The listing builds one solid part. Answer for the finished solid, in the listing's coordinates (mm). Face numbers are marked on the shaded views. A direction names the side the tool comes from. Coordinates: 2 decimals unless noted, no trailing zeros. Order: outer loops, then holes, each group sorted by start corner. A loop starts at its lowest first (then second) coordinate and runs counter-clockwise, first axis right, second up. Notation, with made-up numbers: M 58,42 L 95,42 A34 cw 95,74 Z; hole C 1,56 d9. An arc over 180 degrees is marked long. One line per item, written item: value. Start each with the question number.
Q1. The part is cut by section B-B on z = -55. Give the vertices of the cut face in (x, y), then the cut area to 3 significant figures.
Q2. Each of these flat-tipped pins is pushed along its axis until it touches: pin 1 Ø1.5 at (x, z) = (142.5, -13.5) entering from +Y; pin 2 Ø1.5 at (x, y) = (142.5, -3) entering from -Z; pin 3 Ø2.5 at (x, y) = (142.5, -3) entering from +Z. Where does it stop, or does it pass through?
Q3. The part is cut by section A-A on x = 144. Give the vertices of the cut face in (y, z), then the cut area to 3 significant figures.
Q4. Straight lines are drawn through the part: line 1 along Z through (x, y) = (141.6, -11); line 2 along Y through (x, z) = (141.25, -58); line 3 along Y through (x, z) = (144.05, -38). For each, find the intervals that lie inside material, in ascending order. Write a range as [from, to].
Q5. The part is cut by section C-C on y = -40. Give the vertices of the cut face in (x, z), then the cut area to 3 significant figures.
Q6. For the marked faces 1, 2 and 3, determine the directions among +Z, -Z, +X, -X, +Y, -Y from which every point of the face is accessible in a straight line to the end or side of a thin tool.
```python
from build123d import *

# Parameters (mm, degrees)
BODY_MOVE_COPY1_START         = -65
BODY_MOVE_COPY1_OUTLINE_W     = 5.1
BODY_MOVE_COPY1_OUTLINE_H     = 30.1
BODY_MOVE_COPY1_OUTLINE_R     = 2.6
BODY_MOVE_COPY1_OUTLINE_R_2   = 3.1
BODY_MOVE_COPY1_OUTLINE_R_3   = 1.55
BODY_MOVE_COPY1_OUTLINE_W_2   = 30.5
BODY_MOVE_COPY1_OUTLINE_H_2   = 14.5
BODY_MOVE_COPY1_DEPTH         = 5
BODY_MOVE_COPY1_START_2       = -5
BODY_MOVE_COPY1_2_OUTLINE_W   = 10
BODY_MOVE_COPY1_2_OUTLINE_H   = 5.2
BODY_MOVE_COPY1_2_OUTLINE_R   = 1.6
BODY_MOVE_COPY1_2_OUTLINE_W_2 = 5.1
BODY_MOVE_COPY1_2_OUTLINE_H_2 = 30.1
BODY_MOVE_COPY1_2_DEPTH       = 5
BOSS_EXTRUDE2_DEPTH           = 5


# Read off the part's stored shape, not the designer's step: Body-Move/Copy1
with BuildPart() as part:
    # Body-Move/Copy1 outline → Body-Move/Copy1 (new body)
    with BuildSketch(Plane.XY.offset(BODY_MOVE_COPY1_START)):
        Polygon((24.9, -310), (24.9, -305), (100.2, -305), (100.2, -310), (150, -310), (150, -5), (10.65, -5), (10.65, 0), (-10.65, 0), (-10.65, -5), (-150, -5), (-150, -310), (-100.2, -310), (-100.2, -305), (-24.9, -305), (-24.9, -310), align=None)
        with Locations((-143.45, -280)):
            Rectangle(BODY_MOVE_COPY1_OUTLINE_W, BODY_MOVE_COPY1_OUTLINE_H, mode=Mode.SUBTRACT)
        with Locations((-90, -157.5)):
            Circle(BODY_MOVE_COPY1_OUTLINE_R, mode=Mode.SUBTRACT)
        with Locations((-60, -157.5)):
            Circle(BODY_MOVE_COPY1_OUTLINE_R, mode=Mode.SUBTRACT)
        with Locations((143.45, -280)):
            Rectangle(BODY_MOVE_COPY1_OUTLINE_W, BODY_MOVE_COPY1_OUTLINE_H, mode=Mode.SUBTRACT)
        with Locations((65, -157.5)):
            Circle(BODY_MOVE_COPY1_OUTLINE_R_2, mode=Mode.SUBTRACT)
        with Locations((85, -157.5)):
            Circle(BODY_MOVE_COPY1_OUTLINE_R_2, mode=Mode.SUBTRACT)
        with Locations((-90, -137.5)):
            Circle(BODY_MOVE_COPY1_OUTLINE_R_3, mode=Mode.SUBTRACT)
        with Locations((-60, -137.5)):
            Circle(BODY_MOVE_COPY1_OUTLINE_R_3, mode=Mode.SUBTRACT)
        with Locations((-75, -100.25)):
            Rectangle(BODY_MOVE_COPY1_OUTLINE_W_2, BODY_MOVE_COPY1_OUTLINE_H_2, mode=Mode.SUBTRACT)
        with Locations((-143.45, -30)):
            Rectangle(BODY_MOVE_COPY1_OUTLINE_W, BODY_MOVE_COPY1_OUTLINE_H, mode=Mode.SUBTRACT)
        with Locations((143.45, -30)):
            Rectangle(BODY_MOVE_COPY1_OUTLINE_W, BODY_MOVE_COPY1_OUTLINE_H, mode=Mode.SUBTRACT)
    extrude(amount=BODY_MOVE_COPY1_DEPTH)


with BuildPart() as body_2:
    # Body-Move_Copy1 2 outline → Body-Move_Copy1 2 (new body)
    with BuildSketch(Plane(origin=(0, 0, 0), x_dir=(1, 0, 0), z_dir=(0, 1, 0)).offset(BODY_MOVE_COPY1_START_2)):
        with BuildLine():
            ThreePointArc((-95, -65), (-93.535533906, -61.464466094), (-90, -60))
            Line((-90, -60), (90, -60))
            ThreePointArc((90, -60), (93.535533906, -61.464466094), (95, -65))
            Line((95, -65), (95, -70))
            ThreePointArc((95, -70), (96.464466094, -73.535533906), (100, -75))
            Line((100, -75), (115, -75))
            ThreePointArc((115, -75), (118.535533906, -73.535533906), (120, -70))
            Line((120, -70), (120, -60))
            Line((120, -60), (145.606601718, -34.393398282))
            ThreePointArc((145.606601718, -34.393398282), (148.858192988, -29.52704805), (150, -23.786796564))
            Line((150, -23.786796564), (150, 65))
            Line((150, 65), (10.75, 65))
            Line((10.75, 65), (10.75, 60))
            Line((10.75, 60), (-10.75, 60))
            Line((-10.75, 60), (-10.75, 65))
            Line((-10.75, 65), (-150, 65))
            Line((-150, 65), (-150, -23.786796564))
            ThreePointArc((-150, -23.786796564), (-148.858192988, -29.52704805), (-145.606601718, -34.393398282))
            Line((-145.606601718, -34.393398282), (-120, -60))
            Line((-120, -60), (-120, -70))
            ThreePointArc((-120, -70), (-118.535533906, -73.535533906), (-115, -75))
            Line((-115, -75), (-100, -75))
            ThreePointArc((-100, -75), (-96.464466094, -73.535533906), (-95, -70))
            Line((-95, -70), (-95, -65))
        make_face()
        with Locations((-107.5, -67.5)):
            Rectangle(BODY_MOVE_COPY1_2_OUTLINE_W, BODY_MOVE_COPY1_2_OUTLINE_H, mode=Mode.SUBTRACT)
        with Locations((-110, -52.5)):
            Circle(BODY_MOVE_COPY1_2_OUTLINE_R, mode=Mode.SUBTRACT)
        with Locations((-5, -52.5)):
            Circle(BODY_MOVE_COPY1_2_OUTLINE_R, mode=Mode.SUBTRACT)
        with Locations((5, -52.5)):
            Circle(BODY_MOVE_COPY1_2_OUTLINE_R, mode=Mode.SUBTRACT)
        with Locations((107.5, -67.5)):
            Rectangle(BODY_MOVE_COPY1_2_OUTLINE_W, BODY_MOVE_COPY1_2_OUTLINE_H, mode=Mode.SUBTRACT)
        with Locations((110, -52.5)):
            Circle(BODY_MOVE_COPY1_2_OUTLINE_R, mode=Mode.SUBTRACT)
        with Locations((-143.45, 35)):
            Rectangle(BODY_MOVE_COPY1_2_OUTLINE_W_2, BODY_MOVE_COPY1_2_OUTLINE_H_2, mode=Mode.SUBTRACT)
        with Locations((-110, 52.5)):
            Circle(BODY_MOVE_COPY1_2_OUTLINE_R, mode=Mode.SUBTRACT)
        with Locations((-5, 52.5)):
            Circle(BODY_MOVE_COPY1_2_OUTLINE_R, mode=Mode.SUBTRACT)
        with BuildLine():
            Line((131.606601718, -30.178932188), (115.267766953, -46.517766953))
            ThreePointArc((115.267766953, -46.517766953), (114.456708581, -47.059698831), (113.5, -47.25))
            Line((113.5, -47.25), (107.75, -47.25))
            ThreePointArc((107.75, -47.25), (105.982233047, -47.982233047), (105.25, -49.75))
            Line((105.25, -49.75), (105.25, -53.5))
            ThreePointArc((105.25, -53.5), (104.517766953, -55.267766953), (102.75, -56))
            Line((102.75, -56), (13.25, -56))
            ThreePointArc((13.25, -56), (11.482233047, -55.267766953), (10.75, -53.5))
            Line((10.75, -53.5), (10.75, -49.75))
            ThreePointArc((10.75, -49.75), (10.017766953, -47.982233047), (8.25, -47.25))
            Line((8.25, -47.25), (-8.25, -47.25))
            ThreePointArc((-8.25, -47.25), (-10.017766953, -47.982233047), (-10.75, -49.75))
            Line((-10.75, -49.75), (-10.75, -53.5))
            ThreePointArc((-10.75, -53.5), (-11.482233047, -55.267766953), (-13.25, -56))
            Line((-13.25, -56), (-102.75, -56))
            ThreePointArc((-102.75, -56), (-104.517766953, -55.267766953), (-105.25, -53.5))
            Line((-105.25, -53.5), (-105.25, -49.75))
            ThreePointArc((-105.25, -49.75), (-105.982233047, -47.982233047), (-107.75, -47.25))
            Line((-107.75, -47.25), (-113.5, -47.25))
            ThreePointArc((-113.5, -47.25), (-115.267766953, -46.517766953), (-116, -44.75))
            Line((-116, -44.75), (-116, 44.75))
            ThreePointArc((-116, 44.75), (-115.267766953, 46.517766953), (-113.5, 47.25))
            Line((-113.5, 47.25), (-107.75, 47.25))
            ThreePointArc((-107.75, 47.25), (-105.982233047, 47.982233047), (-105.25, 49.75))
            Line((-105.25, 49.75), (-105.25, 53.5))
            ThreePointArc((-105.25, 53.5), (-104.517766953, 55.267766953), (-102.75, 56))
            Line((-102.75, 56), (-13.25, 56))
            ThreePointArc((-13.25, 56), (-11.482233047, 55.267766953), (-10.75, 53.5))
            Line((-10.75, 53.5), (-10.75, 49.75))
            ThreePointArc((-10.75, 49.75), (-10.017766953, 47.982233047), (-8.25, 47.25))
            Line((-8.25, 47.25), (8.25, 47.25))
            ThreePointArc((8.25, 47.25), (10.017766953, 47.982233047), (10.75, 49.75))
            Line((10.75, 49.75), (10.75, 53.5))
            ThreePointArc((10.75, 53.5), (11.482233047, 55.267766953), (13.25, 56))
            Line((13.25, 56), (102.75, 56))
            ThreePointArc((102.75, 56), (104.517766953, 55.267766953), (105.25, 53.5))
            Line((105.25, 53.5), (105.25, 49.75))
            ThreePointArc((105.25, 49.75), (105.982233047, 47.982233047), (107.75, 47.25))
            Line((107.75, 47.25), (113.5, 47.25))
            ThreePointArc((113.5, 47.25), (115.267766953, 47.982233047), (116, 49.75))
            Line((116, 49.75), (116, 53.5))
            ThreePointArc((116, 53.5), (116.732233047, 55.267766953), (118.5, 56))
            Line((118.5, 56), (133.5, 56))
            ThreePointArc((133.5, 56), (135.267766953, 55.267766953), (136, 53.5))
            Line((136, 53.5), (136, -19.57233047))
            ThreePointArc((136, -19.57233047), (134.858192988, -25.312581956), (131.606601718, -30.178932188))
        make_face(mode=Mode.SUBTRACT)
        with Locations((5, 52.5)):
            Circle(BODY_MOVE_COPY1_2_OUTLINE_R, mode=Mode.SUBTRACT)
        with Locations((143.45, 35)):
            Rectangle(BODY_MOVE_COPY1_2_OUTLINE_W_2, BODY_MOVE_COPY1_2_OUTLINE_H_2, mode=Mode.SUBTRACT)
        with Locations((110, 52.5)):
            Circle(BODY_MOVE_COPY1_2_OUTLINE_R, mode=Mode.SUBTRACT)
    extrude(amount=BODY_MOVE_COPY1_2_DEPTH)


with BuildPart() as body_3:
    # Sketch18 → Boss-Extrude2 (new body)
    with BuildSketch(Plane(origin=(140.9, 0, 0), x_dir=(0, 0, -1), z_dir=(1, 0, 0))):
        with BuildLine():
            Line((20.05, 0), (20.05, -5))
            Line((20.05, -5), (9.95, -5))
            Line((9.95, -5), (9.95, -12.376406871))
            ThreePointArc((9.95, -12.376406871), (11.091807012, -18.116658357), (14.343398282, -22.983008589))
            Line((14.343398282, -22.983008589), (42.016991411, -50.656601718))
            ThreePointArc((42.016991411, -50.656601718), (46.883341643, -53.908192988), (52.623593129, -55.05))
            Line((52.623593129, -55.05), (60, -55.05))
            Line((60, -55.05), (60, -44.95))
            Line((60, -44.95), (65, -44.95))
            Line((65, -44.95), (65, -15.05))
            Line((65, -15.05), (60, -15.05))
            Line((60, -15.05), (60, -7))
            ThreePointArc((60, -7), (59.414213562, -5.585786438), (58, -5))
            Line((58, -5), (49.95, -5))
            Line((49.95, -5), (49.95, 0))
            Line((49.95, 0), (20.05, 0))
        make_face()
    extrude(amount=BOSS_EXTRUDE2_DEPTH)


solid = body_3.part
```
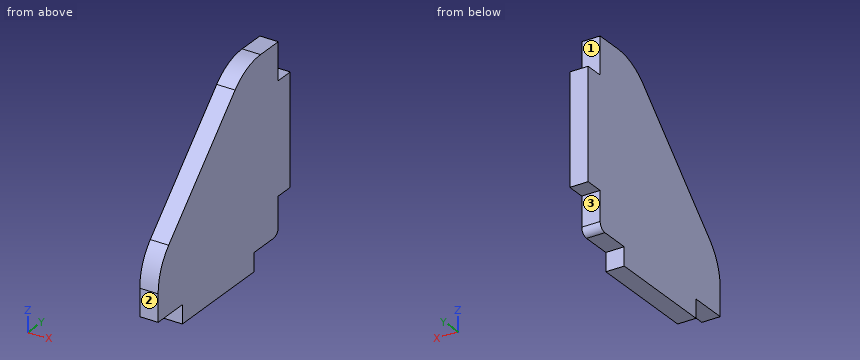
Output:
1. outline: M 140.9,-55.05 L 145.9,-55.05 L 145.9,-5 L 140.9,-5 Z
1. area: 250 mm^2
2. pin 1: stops at y = -5
2. pin 2: stops at z = -49.95
2. pin 3: stops at z = -20.05
3. outline: M -55.05,-60 L -44.95,-60 L -44.95,-65 L -15.05,-65 L -15.05,-60 L -7,-60 A2 ccw -5,-58 L -5,-49.95 L 0,-49.95 L 0,-20.05 L -5,-20.05 L -5,-9.95 L -12.38,-9.95 A15 ccw -22.98,-14.34 L -50.66,-42.02 A15 ccw -55.05,-52.62 Z
3. area: 2,130 mm^2
4. line 1: z = [-60, -9.95]
4. line 2: y = [-55.05, -5]
4. line 3: y = [-46.64, 0]
5. outline: M 140.9,-65 L 145.9,-65 L 145.9,-31.36 L 140.9,-31.36 Z
5. area: 168 mm^2
6. face 1: +Z, +X, -X, +Y
6. face 2: +Z, -Z, +X, -X, -Y
6. face 3: -Z, +X, -X, +Y
